For this review, take the finished solid that the model builds, in its own axes (mm). Face numbers are marked on the shaded views. A direction names the side the tool comes from. Give positions to 0.01 mm unless a question says otherwise; leave off trailing zeros. Order: outer loops, then holes, each group sorted by start corner. A loop starts at its lowest first (then second) coordinate and runs counter-clockwise, first axis right, second up. Notation, with made-up numbers: (-2, -28.5) -> (22, -28.5) arc R24 cw to (22, -15.5) -> close; hole circle Ø5 at (62.25, -3). An arc over 180 degrees is marked (long way). Use CSV: the item, a comma, the result in double quotes. Start each with the question number.
```python
from build123d import *

# Parameters (mm, degrees)
CROQUIS1_R                   = 1.5
SALIENTE_EXTRUIR1_DEPTH      = 10.7
SALIENTE_EXTRUIR2_DEPTH      = 0.0001
SALIENTE_EXTRUIR2_DEPTH_BACK = 0.8
CROQUIS2_R                   = 2.825
CHAFL_N1_SIZE                = 0.8
CROQUIS3_R                   = 1.05
CORTAR_EXTRUIR1_DEPTH        = 10.4
REDONDEO2_R                  = 0.8
CROQUIS6_W                   = 3
CROQUIS6_H                   = 0.4
CORTAR_EXTRUIR4_DEPTH        = 3.5


with BuildPart() as part:
    # Croquis1 → Saliente-Extruir1 (new body)
    with BuildSketch(Plane(origin=(0, 0, 0), x_dir=(1, 0, 0), z_dir=(0, 1, 0))):
        with Locations(Location((0, 0, 0), (0, 0, 270))):
            Circle(CROQUIS1_R)
    extrude(amount=SALIENTE_EXTRUIR1_DEPTH)

    # Croquis2 → Saliente-Extruir2 (add, two sides: drawn at the far end of the back side and taken through both)
    with BuildSketch(Plane(origin=(0, 10.7, 0), x_dir=(1, 0, 0), z_dir=(0, 1, 0)).offset(-SALIENTE_EXTRUIR2_DEPTH_BACK)):
        with Locations(Location((0, 0, 0), (0, 0, 270))):
            Circle(CROQUIS2_R)
    extrude(amount=SALIENTE_EXTRUIR2_DEPTH + SALIENTE_EXTRUIR2_DEPTH_BACK)

    # Chaflán1
    chafl_n1_edges = [part.edges().sort_by_distance(p)[0] for p in [
        (0, 10.7001, -2.825),
    ]]
    chamfer(chafl_n1_edges, length=CHAFL_N1_SIZE)

    # Croquis3 → Cortar-Extruir1 (cut)
    with BuildSketch(Plane(origin=(0, 10.7001, 0), x_dir=(1, 0, 0), z_dir=(0, 1, 0))):
        with Locations(Location((0, 0, 0), (0, 0, 270))):
            Circle(CROQUIS3_R)
    extrude(amount=-CORTAR_EXTRUIR1_DEPTH, mode=Mode.SUBTRACT)

    # Redondeo2
    redondeo2_edges = [part.edges().sort_by_distance(p)[0] for p in [
        (0, 0.3001, -1.05),
    ]]
    fillet(redondeo2_edges, radius=REDONDEO2_R)

    # Croquis6 → Cortar-Extruir4 (cut)
    with BuildSketch(Plane(origin=(0, 0, 0), x_dir=(-1, 0, 0), z_dir=(0, -1, 0))):
        Rectangle(CROQUIS6_W, CROQUIS6_H)
    extrude(amount=-CORTAR_EXTRUIR4_DEPTH, mode=Mode.SUBTRACT)


solid = part.part
```
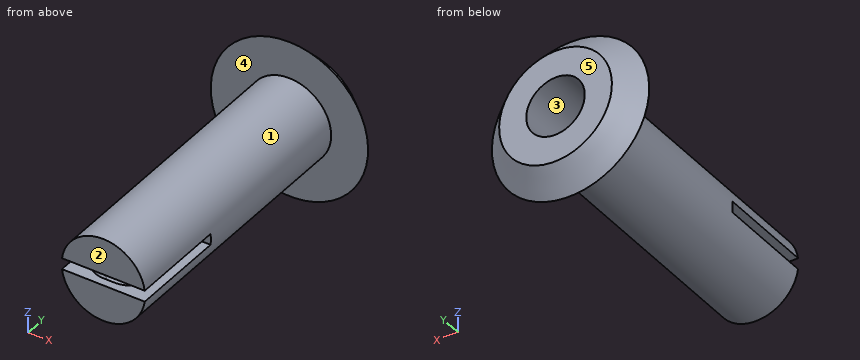
1. For the marked faces 4 and 5, list the 3-axis set-ups (+Z, -Z, +X, -X, +Y, -Y) from which the entire face can be reached by the end or side of a thin tool; tool diameter is ignored.
2. Consider section C-C (y = 9.5). State the section outline as (x, z) points.
3. Draft analysis for pull direction X (two halves, no side actions). For the marked faces 1, 2 and 3, state which applies: +X half, -X half, draft (parallel to the pull), parting line (faces both ways), or undercut.
4. Clearance check with flat-ended pins moving along their axes: P1, Ø2.5, axis at x = -0.5, y = 1, coming from the -Z side; P2, Ø1, axis at y = 7.5, z = 0, coming from the -X side; P3, Ø2, axis at x = -1, y = 1.5, coming from the +Z side. State where each tip first meets the part, or that it passes through.
5. To check wall thickness, follow L1, parallel to X at y = 7.75, z = 0; L2, parallel to Z at x = 0.15, y = 10. State the ranges of each line that lie inside material, in increasing order. Write a range as [from, to].
Answer list:
1,face 4,"-Y"
1,face 5,"+Z, -Z, +X, -X, +Y"
2,outline,"circle Ø3 at (0, 0); hole circle Ø2.1 at (0, 0)"
3,face 1,"parting line"
3,face 2,"draft"
3,face 3,"undercut"
4,P1,"z = -1.5"
4,P2,"x = -1.5"
4,P3,"z = 1.5"
5,L1,"[-1.5, -1.05], [1.05, 1.5]"
5,L2,"[-2.72, -1.04], [1.04, 2.72]"
